Model file for the job. Use its own axes, mm. A direction names the side the tool comes from. Give positions to 0.01 mm unless a question says otherwise; leave off trailing zeros. Loops run counter-clockwise (first coordinate to the right, second up) from the corner with the lowest first, then second, coordinate; pieces in that order, holes last. Notation, with made-up numbers: M 62.5,-13 L 119.5,-13 A12 ccw 119.5,-4 Z; hole C 76.5,-23.75 d3. An arc over 180 degrees is marked long. Answer in a Markdown table with one row per item.
```python
from build123d import *

# Parameters (mm, degrees)
SKETCH1_R           = 3.175
BOSS_EXTRUDE1_DEPTH = 69.85
BOSS_EXTRUDE2_START = -2.54
BOSS_EXTRUDE2_DEPTH = 2.54


with BuildPart() as part:
    # Sketch1 → Boss-Extrude1 (new body)
    with BuildSketch(Plane(origin=(0, 0, 0), x_dir=(1, 0, 0), z_dir=(0, 1, 0))):
        with Locations(Location((0, 0, 0), (0, 0, 270))):
            Circle(SKETCH1_R)
    extrude(amount=BOSS_EXTRUDE1_DEPTH)

    # Sketch2 → Boss-Extrude2 (add)
    with BuildSketch(Plane(origin=(0, 69.85, 0), x_dir=(1, 0, 0), z_dir=(0, 1, 0)).offset(BOSS_EXTRUDE2_START)):
        with BuildLine():
            Line((1.27, 4.259709497), (1.27, 2.909935566))
            ThreePointArc((1.27, 2.909935566), (0, 3.175), (-1.27, 2.909935566))
            Line((-1.27, 2.909935566), (-1.27, 4.259709497))
            ThreePointArc((-1.27, 4.259709497), (0, 4.445), (1.27, 4.259709497))
        make_face()
    extrude(amount=BOSS_EXTRUDE2_DEPTH)


solid = part.part
```
Q1. Drop flat-ended pins along their axis: pin 1 (1.5 mm diameter, centred on x = -0.5, y = 48, fed in from -Z) (3 decimals); pin 2 (1.5 mm diameter, centred on y = 69, z = -3.5, fed in from +X); pin 3 (1 mm diameter, centred on x = 1.5, y = 47, fed in from +Z). Give the stop position or say it passes through.
Reported:
| item | result |
|---|---|
| pin 1 | z = -3.175 |
| pin 2 | x = 1.59 |
| pin 3 | z = 3.01 |
Q2. Saw through at A-A (x = 0). Give the cut face in (y, z) (3 decimals).
Reported:
| item | result |
|---|---|
| outline | M 0,-3.175 L 67.31,-3.175 L 67.31,-4.445 L 69.85,-4.445 L 69.85,3.175 L 0,3.175 Z |
Q3. Saw through at D-D (z = 2.5). Give the cut face in (x, y).
Reported:
| item | result |
|---|---|
| outline | M -1.96,0 L 1.96,0 L 1.96,69.85 L -1.96,69.85 Z |
Q4. Saw through at B-B (y = 17). Give the cut face in (x, z) (3 decimals), and give its area (3 significant figures).
Reported:
| item | result |
|---|---|
| outline | C 0,0 d6.35 |
| area | 31.7 mm² |
Q5. Saw through at C-C (z = -1). Give the cut face in (x, y).
Reported:
| item | result |
|---|---|
| outline | M -3.01,0 L 3.01,0 L 3.01,69.85 L -3.01,69.85 Z |
Q6. 3-axis set-ups, long thin cutter, end or side, ignore diameter. For faces 1 (the face through (-0.018, 68.562, -4.445)), 2 (the face through (1.27, 69, -4)), 3 (the face through (-1.27, 69, -4)): which of +Z, -Z, +X, -X, +Y, -Y reach the whole face in a straight line?
Reported:
| item | result |
|---|---|
| face 1 | -Z, +Y, -Y |
| face 2 | -Z, +X, +Y, -Y |
| face 3 | -Z, -X, +Y, -Y |
Q7. Probe probe 1 along Z at (x, y) = (0, 63) (3 decimals); probe 2 along Y at (x, z) = (1, -3.25); probe 3 along Z at (x, y) = (0.75, 62.5). List the from-to ranges inside material, lowest first.
Reported:
| item | result |
|---|---|
| probe 1 | -3.175 to 3.175 |
| probe 2 | 67.31 to 69.85 |
| probe 3 | -3.09 to 3.09 |
